```python
from build123d import *

# Parameters (mm, degrees)
BOSS_EXTRUDE1_DEPTH = 6
M5_TAPPED_HOLE1_D   = 4.2
FILLET1_R           = 3
FILLET2_R           = 0.5
FILLET3_R           = 0.25


with BuildPart() as part:
    # Sketch1 → Boss-Extrude1 (new body)
    with BuildSketch(Plane.XY):
        Polygon((3.1, 0), (-3.1, 0), (-3.1, -0.5), (-5, -0.5), (-5, -2), (-3, -4), (3, -4), (5, -2), (5, -0.5), (3.1, -0.5), align=None)
    extrude(amount=BOSS_EXTRUDE1_DEPTH)

    # M5 Tapped Hole1 (through all)
    with Locations(Plane(origin=(0, 0, 0), x_dir=(-1, 0, 0), z_dir=(0, 1, 0))):
        with Locations((0, 3)):
            Hole(M5_TAPPED_HOLE1_D / 2)

    # Fillet1
    fillet1_edges = [part.edges().sort_by_distance(p)[0] for p in [
        (-3.1, -0.25, 0),
        (3.1, -0.25, 6),
    ]]
    fillet(fillet1_edges, radius=FILLET1_R)

    # Fillet2
    fillet2_edges = [part.edges().sort_by_distance(p)[0] for p in [
        (5, -2, 3),
        (3, -4, 3),
        (-3, -4, 3),
        (-5, -2, 3),
    ]]
    fillet(fillet2_edges, radius=FILLET2_R)

    # Fillet3
    fillet3_edges = [part.edges().sort_by_distance(p)[0] for p in [
        (-5, -1.146446609, 6),
        (-5, -1.146446609, 0),
        (5, -1.146446609, 0),
        (5, -1.146446609, 6),
        (4, -3, 0),
        (0, -4, 0),
        (-4, -3, 0),
        (-2.984234935, -3.961939766, 0),
        (-4.961939766, -1.984234935, 0),
        (2.984234935, -3.961939766, 0),
        (4.961939766, -1.984234935, 0),
        (4, -3, 6),
        (-4, -3, 6),
        (0, -4, 6),
        (-2.984234935, -3.961939766, 6),
        (-4.961939766, -1.984234935, 6),
        (2.984234935, -3.961939766, 6),
        (4.961939766, -1.984234935, 6),
    ]]
    fillet(fillet3_edges, radius=FILLET3_R)


solid = part.part
```
Verification items for the finished model (mm, model axes). A direction names the side the tool comes from. Coordinates: 2 decimals unless noted, no trailing zeros. Write each loop counter-clockwise with the first axis right and the second up, starting at its lowest first coordinate (ties: lowest second). Pieces come first, ordered by that corner, then holes. Notation, with made-up numbers: (-21.5, 76) - (16.5, 76) arc R17 ccw to (16.5, 91) - close; hole circle Ø2 at (48.5, 85). An arc over 180 degrees is marked (long way). Write item = value, one per line.
Q1. Material ranges on L1, parallel to Z at x = 0, y = -0.85; L2, parallel to Z at x = 1, y = -2.65; L3, parallel to X at y = -2.05, z = 3.25, recorded low to high. Write a range as from..to.
Answer:
L1 = 0..0.9, 5.1..6
L2 = 0..1.15, 4.85..6
L3 = -4.93..-2.09, 2.09..4.93
Q2. Cross-section at B-B (x = 0). Enter the section's corners in (y, z).
Answer:
outline = (-4, 0.25) arc R0.25 ccw to (-3.75, 0) - (0, 0) - (0, 0.9) - (-4, 0.9) - close; (-4, 5.1) - (0, 5.1) - (0, 6) - (-3.75, 6) arc R0.25 ccw to (-4, 5.75) - close
Q3. Cross-section at A-A (z = 4.5). Enter the section's corners in (x, y), plus the area to 3 significant figures.
Answer:
outline = (-5, -1.79) arc R0.5 ccw to (-4.85, -2.15) - (-3.15, -3.85) arc R0.5 ccw to (-2.79, -4) - (-1.47, -4) - (-1.47, 0) - (-3.1, 0) - (-3.1, -0.5) - (-5, -0.5) - close; (1.47, -4) - (2.79, -4) arc R0.5 ccw to (3.15, -3.85) - (4.85, -2.15) arc R0.5 ccw to (5, -1.79) - (5, -0.5) - (2.7, -0.5) - (2.7, 0) - (1.47, 0) - close
area = 22.1 mm²
Q4. Cross-section at D-D (z = 1.25). Enter the section's corners in (x, y).
Answer:
outline = (-5, -1.79) arc R0.5 ccw to (-4.85, -2.15) - (-3.15, -3.85) arc R0.5 ccw to (-2.79, -4) - (-1.16, -4) - (-1.16, 0) - (-2.54, 0) - (-2.54, -0.5) - (-5, -0.5) - close; (1.16, -4) - (2.79, -4) arc R0.5 ccw to (3.15, -3.85) - (4.85, -2.15) arc R0.5 ccw to (5, -1.79) - (5, -0.5) - (3.1, -0.5) - (3.1, 0) - (1.16, 0) - close
Q5. Mould release check, pull along Z, two halves, no side actions. Record for faces 1 (the face through (2.24, -0.25, 5.1)), 2 (the face through (-5, -1, 3)), 3 (the face through (-0.46, -2.03, 0.95)): released by +Z, released by -Z, zero draft, split by the parting line, or undercut.
Answer:
face_1 = released by +Z
face_2 = zero draft
face_3 = undercut
Q6. Cross-section at C-C (y = -0.3). Enter the section's corners in (x, z).
Answer:
outline = (-3.1, 3) arc R3 ccw to (-0.1, 0) - (3.1, 0) - (3.1, 3) arc R3 ccw to (0.1, 6) - (-3.1, 6) - close; hole circle Ø4.2 at (0, 3)
Q7. Access from +Z, -Z, +X, -X, +Y, -Y to the whole of each face (thin tool, end or side, straight path). Record for faces 4 (the face through (-4, -3, 3)), 5 (the face through (-2.2, -0.25, 0.86)).
Answer:
face_4 = +Z, -Z, -X, -Y
face_5 = -Z, -X, +Y
Q8. Go/stop test with flat-tipped pins: pin 1 Ø1.5 at (y, z) = (-2, 5.5) entering from -X; pin 2 Ø1 at (y, z) = (-2.5, 2.5) entering from +X. Record where each tip stops, or that it passes through.
Answer:
pin_1 = -5
pin_2 = 4.96
